from build123d import *
from build123d.topology import SkipClean

# Parameters (mm, degrees)
EXTRUDE_1_DEPTH          = 10
SKETCH_2_R               = 14
EXTRUDE_2_DEPTH          = 95
EXTRUDE_START            = 9.1
SKETCH_3_R               = 14
EXTRUDE_3_DEPTH          = 9.1
SKETCH_5_R               = 14
EXTRUDE_4_DEPTH          = 9.5
CUT_EXTRUDE_1_DEPTH      = 211.390033392
CUT_EXTRUDE_1_DEPTH_BACK = 211.390033392
SKETCH_6_R               = 5
CUT_EXTRUDE_2_DEPTH      = 19.5


with BuildPart() as part:
    # Sketch 1 → Extrude 1 (new body)
    with BuildSketch(Plane.XY):
        with BuildLine():
            Line((-104.637493626, 39.858490566), (-104.637493626, -55.141509434))
            Line((-104.637493626, -55.141509434), (151.362506374, -55.141509434))
            ThreePointArc((151.362506374, -55.141509434), (176.062506374, -30.441509434), (151.362506374, -5.741509434))
            Line((151.362506374, -5.741509434), (122.362506374, -5.741509434))
            Line((122.362506374, -5.741509434), (-29.637493626, 39.858490566))
            Line((-29.637493626, 39.858490566), (-104.637493626, 39.858490566))
        make_face()
    extrude(amount=EXTRUDE_1_DEPTH)

    # Sketch 2 → Extrude 2 (add)
    with BuildSketch(Plane(origin=(0, 39.858490566, 0), x_dir=(1, 0, 0), z_dir=(0, 1, 0))):
        with Locations((-90.637493626, -5)):
            Circle(SKETCH_2_R)
    extrude(amount=-EXTRUDE_2_DEPTH)

    # Sketch 3 → Extrude 3 (add)
    with BuildSketch(Plane(origin=(0, 39.858490566, 0), x_dir=(1, 0, 0), z_dir=(0, 1, 0)).offset(EXTRUDE_START)):
        with Locations(Location((-90.637493626, -5, 0), (0, 0, 180))):
            Circle(SKETCH_3_R)
    extrude(amount=-EXTRUDE_3_DEPTH)

    # Sketch 5 → Extrude 4 (add)
    with SkipClean():  # the faces are left unmerged after this step: merging them gives an invalid solid
        with BuildSketch(Plane.XZ.offset(55.141509434)):
            with Locations(Location((-90.637493626, 5, 0), (0, 0, 180))):
                Circle(SKETCH_5_R)
        extrude(amount=EXTRUDE_4_DEPTH)
    add(part.part.scale(1), mode=Mode.REPLACE)  # the faces are merged on a copy

    # Sketch 6 → Cut-Extrude 1 (cut, two sides: drawn at the far end of the back side and taken through both)
    with BuildSketch(Plane(origin=(0, 48.958490566, 0), x_dir=(1, 0, 0), z_dir=(0, 1, 0)).offset(-CUT_EXTRUDE_1_DEPTH_BACK)):
        with Locations(Location((-90.637493626, -5, 0), (0, 0, 180))):
            Circle(SKETCH_6_R)
    extrude(amount=CUT_EXTRUDE_1_DEPTH + CUT_EXTRUDE_1_DEPTH_BACK, mode=Mode.SUBTRACT)

    # Sketch 7 → Cut-Extrude 2 (cut)
    with BuildSketch(Plane.XY.offset(10)):
        with BuildLine():
            Line((-77.560796795, 15.329522676), (-66.456337958, 15.329522676))
            ThreePointArc((-66.456337958, 15.329522676), (-62.920804052, 13.865056582), (-61.456337958, 10.329522676))
            Line((-61.456337958, 10.329522676), (-61.456337958, -32.291143793))
            ThreePointArc((-61.456337958, -32.291143793), (-62.920804052, -35.826677699), (-66.456337958, -37.291143793))
            Line((-66.456337958, -37.291143793), (-77.560796795, -37.291143793))
            Line((-77.560796795, -37.291143793), (-77.560796795, 15.329522676))
        make_face()
        with BuildLine():
            Line((-44.713398627, 8.282778838), (-44.713398627, -32.291143793))
            ThreePointArc((-44.713398627, -32.291143793), (-43.248932532, -35.826677699), (-39.713398627, -37.291143793))
            Line((-39.713398627, -37.291143793), (76.245027984, -37.291143793))
            ThreePointArc((76.245027984, -37.291143793), (81.1743885, -33.128642988), (77.896362169, -27.571705753))
            Line((77.896362169, -27.571705753), (-38.062064442, 13.002216878))
            ThreePointArc((-38.062064442, 13.002216878), (-42.606781515, 12.360564446), (-44.713398627, 8.282778838))
        make_face()
    extrude(amount=-CUT_EXTRUDE_2_DEPTH, mode=Mode.SUBTRACT)


solid = part.part
Check sheet for the modelled part. Datum: model origin and axes. Units: mm. A direction names the side the tool comes from. Give positions to 0.01 mm unless a question says otherwise; leave off trailing zeros. Write each loop counter-clockwise with the first axis right and the second up, starting at its lowest first coordinate (ties: lowest second). Pieces come first, ordered by that corner, then holes. Notation, with made-up numbers: (65, 73) -> (123, 73) arc R22 ccw to (123, 93) -> close; hole circle Ø7 at (55.5, 20.5). An arc over 180 degrees is marked (long way). Use one line per item in the form item = value. Start each with the question number.
1. Section check C-C (x = -52.5). Record the cut outline in (y, z), and give its area (3 significant figures).
2. Section check D-D (y = -51.5). Record the cut outline in (x, z), and give its area (3 significant figures).
3. Thickness scan on line 1 along Z through (x, y) = (-23, 15); line 2 along Y through (x, z) = (-11, 1.25); line 3 along Y through (x, z) = (30.5, 3). Record the ranges inside material, lowest first. Write a range as from..to.
4. Section check A-A (x = 52). Record the cut outline in (y, z), and give its area (3 significant figures).
5. Mould release check, pull along Y, two halves, no side actions. Record for faces 3 (the flat face through (137, -5.742, 5)), 4 (the cylindrical face through (-62.96, 13.904, 5.07)), 5 (the flat face through (47, -7, 10)): pulls with the +Y half, pulls with the -Y half, needs draft (parallel to the pull), parting line crosses it, or undercut.
6. Go/stop test with flat-tipped pins: P1, Ø11, axis at x = 26, z = 7, coming from the -Y side; P2, Ø12, axis at x = -76, z = 0.5, coming from the -Y side; P3, Ø8, axis at x = 134, z = 3, coming from the +Y side; P4, Ø3, axis at x = 46, y = -9.5, coming from the +Z side. Record where each tip stops, or that it passes through.
7. Access from +Z, -Z, +X, -X, +Y, -Y to the whole of each face (thin tool, end or side, straight path). Record for faces 1 (the flat face through (47.43, 16.74, 4.93)), 2 (the cylindrical face through (81.157, -33.225, 5.07)).
8. Section check B-B (y = -1). Record the cut outline in (x, z), and give its area (3 significant figures).
Conclusion:
q1.outline = (-55.14, 0) -> (39.86, 0) -> (39.86, 10) -> (-55.14, 10) -> close
q1.area = 950 mm²
q2.outline = (-104.64, 0) -> (-103.71, 0) arc R14 ccw to (-77.56, 0) -> (164.27, 0) -> (164.27, 10) -> (-77.56, 10) arc R14 ccw to (-103.71, 10) -> (-104.64, 10) -> close; hole circle Ø10 at (-90.64, 5)
q2.area = 2,950 mm²
q3.line_1 = 0..10
q3.line_2 = -55.14..-37.29, 3.53..34.27
q3.line_3 = -55.14..-37.29, -10.99..21.82
q4.outline = (-55.14, 0) -> (-37.29, 0) -> (-37.29, 10) -> (-55.14, 10) -> close; (-18.51, 0) -> (15.37, 0) -> (15.37, 10) -> (-18.51, 10) -> close
q4.area = 517 mm²
q5.face_3 = pulls with the +Y half
q5.face_4 = undercut
q5.face_5 = needs draft
q6.P1 = -55.14
q6.P2 = -64.64
q6.P3 = -5.74
q6.P4 = 10
q7.face_1 = +Z, -Z, +X, +Y
q7.face_2 = +Z, -Z
q8.outline = (-104.64, 0) -> (-103.71, 0) arc R14 ccw to (-77.56, 0) -> (-77.56, 10) arc R14 ccw to (-103.71, 10) -> (-104.64, 10) -> close; (-61.46, 0) -> (-44.71, 0) -> (-44.71, 10) -> (-61.46, 10) -> close; (1.96, 0) -> (106.56, 0) -> (106.56, 10) -> (1.96, 10) -> close; hole circle Ø10 at (-90.64, 5)
q8.area = 1,750 mm²
